Geometry: final body of the model. Coordinates: model frame, mm. Face numbers are marked on the shaded views. Coordinates: 2 decimals unless noted, no trailing zeros. Write each loop counter-clockwise with the first axis right and the second up, starting at its lowest first coordinate (ties: lowest second). Pieces come first, ordered by that corner, then holes. Notation, with made-up numbers: (58.25, -26) -> (82.25, -26) arc R35 ccw to (82.25, 9) -> close; hole circle Ø4 at (-34.75, 63.25). An arc over 180 degrees is marked (long way). One line per item, written item: value.
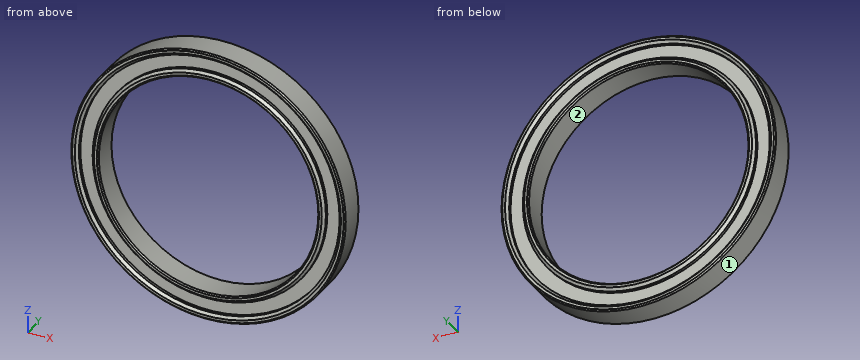
```python
from build123d import *

# Parameters (mm, degrees)
SKETCH1_R           = 50
SKETCH1_R_2         = 40
BOSS_EXTRUDE1_DEPTH = 10
CHAMFER1_SIZE       = 0.5
SKETCH2_R           = 47.5
SKETCH2_R_2         = 42.5
CUT_EXTRUDE1_DEPTH  = 2
CHAMFER2_SIZE       = 1
SKETCH3_R           = 47.5
SKETCH3_R_2         = 42.5
CUT_EXTRUDE2_DEPTH  = 2
CHAMFER3_SIZE       = 1


with BuildPart() as part:
    # Sketch1 → Boss-Extrude1 (new body)
    with BuildSketch(Plane(origin=(0, 0, 0), x_dir=(1, 0, 0), z_dir=(0, 1, 0))):
        Circle(SKETCH1_R)
        Circle(SKETCH1_R_2, mode=Mode.SUBTRACT)
    extrude(amount=BOSS_EXTRUDE1_DEPTH)

    # Chamfer1
    chamfer1_edges = [part.edges().sort_by_distance(p)[0] for p in [
        (-50, 0, 0),
        (-50, 10, 0),
        (-40, 0, 0),
        (-40, 10, 0),
    ]]
    chamfer(chamfer1_edges, length=CHAMFER1_SIZE)

    # Sketch2 → Cut-Extrude1 (cut)
    with BuildSketch(Plane(origin=(0, 10, 0), x_dir=(1, 0, 0), z_dir=(0, 1, 0))):
        Circle(SKETCH2_R)
        Circle(SKETCH2_R_2, mode=Mode.SUBTRACT)
    extrude(amount=-CUT_EXTRUDE1_DEPTH, mode=Mode.SUBTRACT)

    # Chamfer2
    chamfer2_edges = [part.edges().sort_by_distance(p)[0] for p in [
        (-47.5, 10, 0),
        (-42.5, 10, 0),
    ]]
    chamfer(chamfer2_edges, length=CHAMFER2_SIZE)

    # Sketch3 → Cut-Extrude2 (cut)
    with BuildSketch(Plane.XZ):
        Circle(SKETCH3_R)
        Circle(SKETCH3_R_2, mode=Mode.SUBTRACT)
    extrude(amount=-CUT_EXTRUDE2_DEPTH, mode=Mode.SUBTRACT)

    # Chamfer3
    chamfer3_edges = [part.edges().sort_by_distance(p)[0] for p in [
        (-47.5, 0, 0),
        (-42.5, 0, 0),
    ]]
    chamfer(chamfer3_edges, length=CHAMFER3_SIZE)


solid = part.part
```
(1) Pull-direction query (Z, two-part tool) for the marked faces 1 and 2; classes: released by +Z, released by -Z, zero draft, split by the parting line, or undercut.
Responses:
face 1: split by the parting line
face 2: undercut
(2) First-contact query: pin 1 (1.5 mm diameter, centred on x = 31, z = 23.5, fed in from +Y); pin 2 (1 mm diameter, centred on y = 6, z = 39.5, fed in from +X); pin 3 (1 mm diameter, centred on x = -24, y = 4, fed in from -Z); pin 4 (3 mm diameter, centred on y = 2.5, z = 31, fed in from +X). Flat tips, straight axial feed; report the tip coordinate or a pass-through.
Responses:
pin 1: passes through
pin 2: stops at x = 31.29
pin 3: stops at z = -44.13
pin 4: stops at x = 40.37
(3) Section A-A (y = 4.5). Return the cut outline in (x, z), then the cut area to 3 significant figures.
Responses:
outline: circle Ø100 at (0, 0); hole circle Ø80 at (0, 0)
area: 2,830 mm2
(4) Line query: line 1 (Z direction, x = 0, y = 1.55); line 2 (X direction, y = 3.25, z = 0). Output: solid intervals per line, ascending. Write a range as [from, to].
Responses:
line 1: z = [-50, -47.5], [-42.5, -40], [40, 42.5], [47.5, 50]
line 2: x = [-50, -40], [40, 50]
